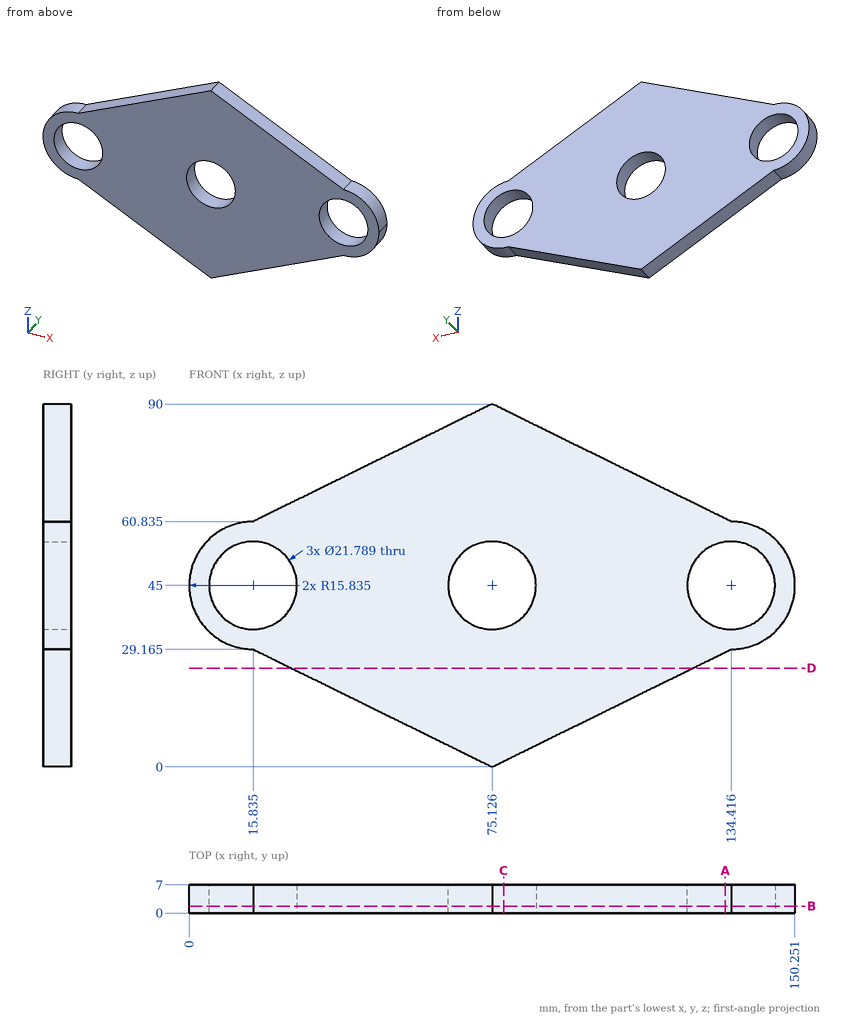
Geometry: see drawing. Coordinates: mm, zero at the bounding-box minimum. Round coordinates to 2 decimals unless told otherwise and drop trailing zeros. Loops run counter-clockwise (first coordinate to the right, second up) from the corner with the lowest first, then second, coordinate; pieces in that order, holes last. Notation, with made-up numbers: (-24, 3) - (18, 3) arc R23 ccw to (18, 29) - close; hole circle Ø7 at (-32.75, -28). An arc over 180 degrees is marked (long way). Write item = value, one per line. Start each with the question number.
(1) Ray query, line 1 along Z through (x, y) = (140.5, 2.5); line 2 along X through (y, z) = (4.5, 54) (1 decimal); line 3 along Z through (x, y) = (16.5, 1.25) (1 decimal). Return the intervals inside material, ascending. Write a range as from..to.
(2) Section query C-C, the plane x = 78. Output: boundary loops of the cut face in (y, z), plus the area to 3 significant figures.
(3) Pin query (flat end, axial travel): pin 1 (2 mm diameter, centred on x = 24, y = 3, fed in from +Z); pin 2 (4 mm diameter, centred on y = 3, z = 24, fed in from +X) (1 decimal); pin 3 (2 mm diameter, centred on x = 104.5, y = 4, fed in from -Z). Return the tip coordinate at first contact, or that it passes through.
(4) Section query A-A, the plane x = 133. Output: boundary loops of the cut face in (y, z).
(5) Section query B-B, the plane y = 1.75. Output: boundary loops of the cut face in (x, z) (1 decimal), plus the area to 3 significant figures.
(6) Section query D-D, the plane z = 24.5. Output: boundary loops of the cut face in (x, y), plus the area to 3 significant figures.
Conclusion:
q1.line_1 = 30.38..35.96, 54.04..59.62
q1.line_2 = 2.8..9.7, 22..69, 81.3..128.3, 140.6..147.4
q1.line_3 = 28.8..34.1, 55.9..61.2
q2.outline = (0, 1.41) - (7, 1.41) - (7, 34.49) - (0, 34.49) - close; (0, 55.51) - (7, 55.51) - (7, 88.59) - (0, 88.59) - close
q2.area = 463 mm2
q3.pin_1 = 65.34
q3.pin_2 = 128
q3.pin_3 = 13.96
q4.outline = (0, 28.47) - (7, 28.47) - (7, 34.2) - (0, 34.2) - close; (0, 55.8) - (7, 55.8) - (7, 61.53) - (0, 61.53) - close
q5.outline = (15.8, 29.2) - (75.1, 0) - (134.4, 29.2) arc R15.8 ccw to (150.3, 45) arc R15.8 ccw to (134.4, 60.8) - (75.1, 90) - (15.8, 60.8) arc R15.8 ccw to start; hole circle Ø21.8 at (15.8, 45); hole circle Ø21.8 at (75.1, 45); hole circle Ø21.8 at (134.4, 45)
q5.area = 6,880 mm2
q6.outline = (25.32, 0) - (124.93, 0) - (124.93, 7) - (25.32, 7) - close
q6.area = 697 mm2
